from build123d import *

# Parameters (mm, degrees)
F0_R     = 12.7
F0_R_2   = 44.45
F1_DEPTH = 6.35


with BuildPart() as f1:
    # F0 (on Right) → F1 (new body)
    with BuildSketch(Plane.YZ):
        with BuildLine():
            ThreePointArc((-76.824834, -27.378873), (-61.23519, -31.10744), (-48.558824, -40.918097))
            ThreePointArc((-48.558824, -40.918097), (-1.818361, -63.47396), (46.136719, -43.630874))
            ThreePointArc((46.136719, -43.630874), (59.347524, -34.564632), (75.117614, -31.731545))
            ThreePointArc((75.117614, -31.731545), (107.95, 0), (75.117614, 31.731545))
            ThreePointArc((75.117614, 31.731545), (59.347524, 34.564632), (46.136719, 43.630874))
            ThreePointArc((46.136719, 43.630874), (-1.818361, 63.47396), (-48.558824, 40.918097))
            ThreePointArc((-48.558824, 40.918097), (-61.23519, 31.10744), (-76.824834, 27.378873))
            ThreePointArc((-76.824834, 27.378873), (-103.586002, 0), (-76.824834, -27.378873))
        make_face()
        with Locations((-76.2, 0)):
            Circle(F0_R, mode=Mode.SUBTRACT)
        Circle(F0_R_2, mode=Mode.SUBTRACT)
        with Locations((76.2, 0)):
            Circle(F0_R, mode=Mode.SUBTRACT)
    extrude(amount=F1_DEPTH)


solid = f1.part
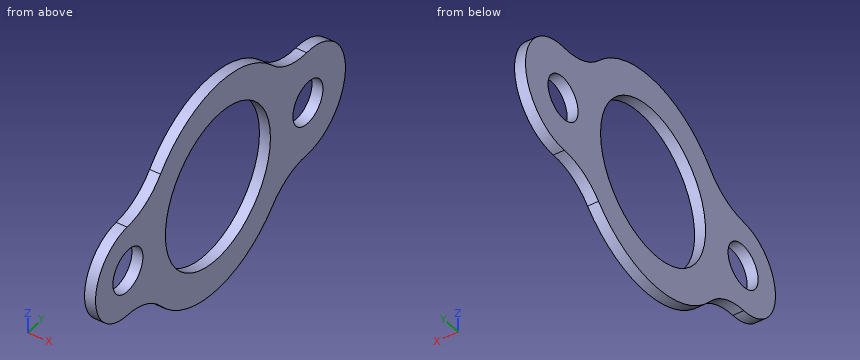
Work out the finished part from the listing and answer in its coordinate system (mm). Give positions to 0.01 mm unless a question says otherwise; leave off trailing zeros. Loops run counter-clockwise (first coordinate to the right, second up) from the corner with the lowest first, then second, coordinate; pieces in that order, holes last. Notation, with made-up numbers: (1.5, -14.5) - (27.5, -14.5) arc R23 cw to (27.5, -1.5) - close; hole circle Ø5 at (12.5, 15). An arc over 180 degrees is marked (long way). Answer in a Markdown table with one row per item.
(1) Consider L1, parallel to Z at x = 4.25, y = 0; L2, parallel to Z at x = 3, y = 76.2; L3, parallel to Y at x = 2, z = 13. Determine where each line is inside the solid, lowest interval first. Write a range as [from, to].
Results list:
| item | result |
|---|---|
| L1 | z = [-63.5, -44.45], [44.45, 63.5] |
| L2 | z = [-31.75, -12.7], [12.7, 31.75] |
| L3 | y = [-100.3, -42.51], [42.51, 105.17] |
(2) Section B-B (z = 0) is taken. Give the vertices of the cut face in (x, y).
Results list:
| item | result |
|---|---|
| outline | (0, -103.59) - (6.35, -103.59) - (6.35, -88.9) - (0, -88.9) - close; (0, -63.5) - (6.35, -63.5) - (6.35, -44.45) - (0, -44.45) - close; (0, 44.45) - (6.35, 44.45) - (6.35, 63.5) - (0, 63.5) - close; (0, 88.9) - (6.35, 88.9) - (6.35, 107.95) - (0, 107.95) - close |
(3) Section C-C (z = 17) is taken. Give the vertices of the cut face in (x, y), and give its area (3 significant figures).
Results list:
| item | result |
|---|---|
| outline | (0, -97.67) - (6.35, -97.67) - (6.35, -41.07) - (0, -41.07) - close; (0, 41.07) - (6.35, 41.07) - (6.35, 103.02) - (0, 103.02) - close |
| area | 753 mm² |
(4) Section D-D (x = 1.75) is taken. Give the vertices of the cut face in (y, z).
Results list:
| item | result |
|---|---|
| outline | (-76.82, -27.38) arc R38.1 cw to (-48.56, -40.92) arc R63.5 ccw to (46.14, -43.63) arc R38.1 cw to (75.12, -31.73) arc R31.75 ccw (long way) to (75.12, 31.73) arc R38.1 cw to (46.14, 43.63) arc R63.5 ccw to (-48.56, 40.92) arc R38.1 cw to (-76.82, 27.38) arc R27.39 ccw to start; hole circle Ø25.4 at (-76.2, 0); hole circle Ø88.9 at (0, 0); hole circle Ø25.4 at (76.2, 0) |
(5) Section A-A (y = 0) is taken. Give the vertices of the cut face in (x, z), and give its area (3 significant figures).
Results list:
| item | result |
|---|---|
| outline | (0, -63.5) - (6.35, -63.5) - (6.35, -44.45) - (0, -44.45) - close; (0, 44.45) - (6.35, 44.45) - (6.35, 63.5) - (0, 63.5) - close |
| area | 242 mm² |
(6) Flat-ended cylindrical pins translate along their axes: pin 1 Ø3 at (x, y) = (1, -67.5) entering from -Z; pin 2 Ø3 at (x, y) = (3.5, 53.5) entering from -Z; pin 3 Ø2 at (x, z) = (5, -10.5) entering from +Y. Find the tip coordinate at first contact, or state that the pin passes through.
Results list:
| item | result |
|---|---|
| pin 1 | stops at z = -29.21 |
| pin 2 | stops at z = -38.58 |
| pin 3 | stops at y = 106.5 |
